Autodesk Inventor part; units mm, degrees
ref_plane "Arbeitsebene1" through (0, 0, 0) normal (0, 0, -1) x (-1, 0, 0)
ref_plane "Arbeitsebene4" through (0, 0, 0) normal (0, 0, -1) x (-1, 0, 0)
ref_plane "Arbeitsebene3" through (-15, 100, 0) normal (0, 1, 0) x (1, 0, 0)
ref_plane "Arbeitsebene1" through (0, 0, 0) normal (0, 0, -1) x (-1, 0, 0)
sketch "Skizze3" plane through (0, 0, 0) normal (0, 0, -1) x (-1, 0, 0)
  point P0 (0, 0)
ref_plane "Arbeitsebene4" through (0, 0, 0) normal (0, 0, -1) x (-1, 0, 0)
sketch "Skizze4" plane through (0, 0, 0) normal (0, 0, -1) x (-1, 0, 0)
  line L0 (15, 68) -> (-15, 68)
  line L1 (-15, 68) -> (-15, 60)
  line L2 (-15, 60) -> (15, 60)
  line L3 (15, 60) -> (15, 68)
  line L4 (-15, 76) -> (15, 76)
  line L5 (15, 76) -> (15, 84)
  line L6 (15, 84) -> (-15, 84)
  line L7 (-15, 84) -> (-15, 76)
  line L8 (-15, 92) -> (15, 92)
  line L9 (15, 92) -> (15, 100)
  line L10 (15, 100) -> (-15, 100)
  line L11 (-15, 100) -> (-15, 92)
  point P0 (0, 0)
  dimension "d7" = 30
  dimension "d8" = 8
  dimension "d9" = 30
  dimension "d10" = 8
  dimension "d11" = 8
extrude "Extrusion3" add sketch "Skizze4" along normal blind 60
ref_plane "Arbeitsebene3" through (-15, 100, 0) normal (0, 1, 0) x (1, 0, 0)
sketch "Skizze5" plane through (-15, 100, 0) normal (0, 1, 0) x (1, 0, 0)
  circle A0 centre (15, 30) radius 7
  line L0 (0, 60) -> (30, 60)
  arc A1 (30, 60) -> (0, 60) centre (15, 60) ccw
  point P0 (15, 0)
  dimension "d14" = 14
  dimension "d15" = 15
extrude "Extrusion4" cut sketch "Skizze5" against normal blind 40 contours A0
sketch "Skizze6" plane through (0, 0, -60) normal (0, 0, -1) x (-1, 0, 0)
  circle A0 centre (0, 80) radius 100
  point P0 (0, 0)
  point P1 (-15, 76)
  dimension "d19" = 200
extrude "Extrusion5" add sketch "Skizze6" along normal blind 30
fillet "Rundung1" radius 2 2 edges at (100, 80, -90) (100, 80, -60)
properties part number "Hochfahren_nach_Stempel"
The listing builds one solid part. Answer for the finished solid, in the listing's coordinates (mm). A direction names the side the tool comes from. Round coordinates to 2 decimals unless told otherwise and drop trailing zeros. Write each loop counter-clockwise with the first axis right and the second up, starting at its lowest first coordinate (ties: lowest second). Pieces come first, ordered by that corner, then holes. Notation, with made-up numbers: (74, 33) - (84, 33) arc R30 cw to (84, 69) - close; hole circle Ø4 at (42, -0.75). An arc over 180 degrees is marked (long way). Use one line per item in the form item = value. Start each with the question number.
Item 1: Determine the mould class of faces 1 (the flat face through (4, 60, -23)), 2 (the flat face through (4, 76, -23)), 3 (the flat face through (-15, 80, -30)), 4 (the flat face through (-4, 68, -23)) for opening direction Y: +Y half, -Y half, draft (parallel to the pull), parting line (faces both ways), or undercut.
Item 2: A cutting plane is placed at B-B (z = -56). Write down the section's boundary in (x, y), plus the area to 3 significant figures.
Item 3: A cutting plane is placed at A-A (x = 0). Give the number of separate pieces and of enclosed holes in the cut face, plus the area to 3 significant figures.
Item 4: A cutting plane is placed at D-D (z = -27.5). Write down the section's boundary in (x, y), plus the area to 3 significant figures.
Item 5: A tool of negligible diameter and unlimited length cuts with its end or side. For faces 5 (the flat face through (-15, 96, -30)), 6 (the flat face through (4, 92, -23)), 7 (the flat face through (-4, 100, -23)), from which of +Z, -Z, +X, -X, +Y, -Y can it reach the whole face along a straight path? Write none if from no direction.
Item 6: Flat-ended cylindrical pins translate along their axes: pin 1 Ø18 at (x, z) = (0, -30) entering from +Y; pin 2 Ø4 at (y, z) = (95.5, -43.5) entering from +X; pin 3 Ø1.5 at (x, y) = (-29.5, 144) entering from +Z. Find the tip coordinate at first contact, or state that the pin passes through.
Item 7: A cutting plane is placed at C-C (y = 80). Write down the section's boundary in (x, z), plus the area to 3 significant figures.
Item 8: Find the intervals of material crossed by line 1 (X direction, y = 61.75, z = -30); line 2 (Z direction, x = 0, y = 66.25); line 3 (Z direction, x = -11, y = 17), in increasing order. Write a range as [from, to].
The answers:
q1.face_1 = -Y half
q1.face_2 = undercut
q1.face_3 = draft
q1.face_4 = undercut
q2.outline = (-15, 60) - (15, 60) - (15, 68) - (-15, 68) - close; (-15, 76) - (15, 76) - (15, 84) - (-15, 84) - close; (-15, 92) - (15, 92) - (15, 100) - (-15, 100) - close
q2.area = 720 mm^2
q3.separate_pieces = 4
q3.enclosed_holes = 0
q3.area = 7,100 mm^2
q4.outline = (-15, 60) - (-6.54, 60) - (-6.54, 68) - (-15, 68) - close; (-15, 76) - (-6.54, 76) - (-6.54, 84) - (-15, 84) - close; (-15, 92) - (-6.54, 92) - (-6.54, 100) - (-15, 100) - close; (6.54, 60) - (15, 60) - (15, 68) - (6.54, 68) - close; (6.54, 76) - (15, 76) - (15, 84) - (6.54, 84) - close; (6.54, 92) - (15, 92) - (15, 100) - (6.54, 100) - close
q4.area = 406 mm^2
q5.face_5 = +Z, -X, +Y, -Y
q5.face_6 = +Z, +X, -X
q5.face_7 = +Z, +X, -X, +Y
q6.pin_1 = 100
q6.pin_2 = 15
q6.pin_3 = -60
q7.outline = (-100, -88) arc R2 ccw to (-98, -90) - (98, -90) arc R2 ccw to (100, -88) - (100, -62) arc R2 ccw to (98, -60) - (15, -60) - (15, 0) - (-15, 0) - (-15, -60) - (-98, -60) arc R2 ccw to (-100, -62) - close; hole circle Ø14 at (0, -30)
q7.area = 7,640 mm^2
q8.line_1 = [-15, -7], [7, 15]
q8.line_2 = [-90, -37], [-23, 0]
q8.line_3 = [-90, -60]
